Part model, mm, in its own coordinate system. Face numbers are marked on the shaded views. A direction names the side the tool comes from. Round coordinates to 2 decimals unless told otherwise and drop trailing zeros. Write each loop counter-clockwise with the first axis right and the second up, starting at its lowest first coordinate (ties: lowest second). Pieces come first, ordered by that corner, then holes.
1) Saw through at D-D on y = -22. Write the cut outline in (x, z) (1 decimal), and give its area (3 significant figures).
2) Saw through at A-A on y = -13. Write the cut outline in (x, z) (3 decimals), and give its area (3 significant figures).
3) Flat gauge pins, fed straight in: pin 1 (12 mm diameter, centred on x = 6, z = 12.5, fed in from +Y); pin 2 (8 mm diameter, centred on x = -4, z = 2, fed in from +Y); pin 3 (13 mm diameter, centred on x = -1, z = 3.5, fed in from +Y); pin 4 (8 mm diameter, centred on x = -6.5, z = -12.5, fed in from -Y). Where does each tip first touch, or does it go through?
4) Which spindle directions (+Z, -Z, +X, -X, +Y, -Y) get a long thin tool onto all of the face, cutting with end or side? Do the marked faces 4, 5 and 6. Say none if no direction does.
5) Drill centre lines: L1, parallel to Z at x = 12, y = 14.5 (3 decimals); L2, parallel to Z at x = 0, y = -28. Where is each one in solid material? Low to high.
6) Pull direction X, two halves, no side cores. Call the marked faces 1, 2 and 3: +X half, -X half, draft (parallel to the pull), parting line (faces both ways), or undercut.
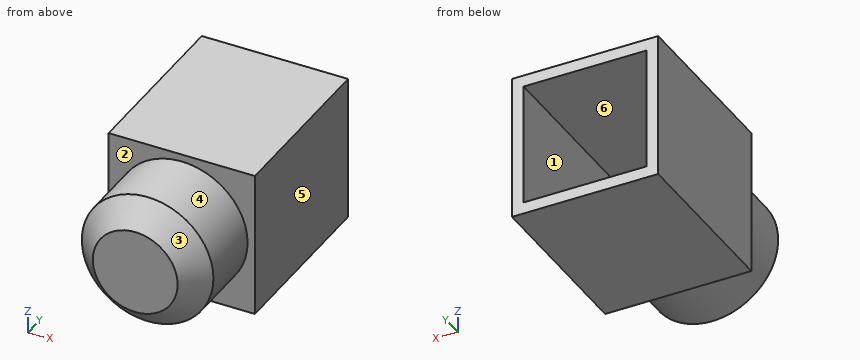
```python
from build123d import *

# Parameters (mm, degrees)
F0_W     = 31.75
F0_H     = 31.75
F1_DEPTH = 19.05
F2_R     = 14.2875
F3_DEPTH = 19.05
F4_SIZE  = 5.08
F5_T     = -2.54


with BuildPart() as f1:
    # F0 (on Front) → F1 (new body, symmetric)
    with BuildSketch(Plane.XZ):
        Rectangle(F0_W, F0_H)
    extrude(amount=F1_DEPTH, both=True)

    # F2 (on face) → F3 (join)
    with BuildSketch(Plane.XZ.offset(19.05)):
        Circle(F2_R)
    extrude(amount=F3_DEPTH)

    # F4
    f4_edges = [f1.edges().sort_by_distance(p)[0] for p in [
        (-14.2875, -38.1, 0),
    ]]
    chamfer(f4_edges, length=F4_SIZE)

    # F5
    f5_openings = [f1.faces().sort_by_distance(p)[0] for p in [
        (0, 19.05, 0),
    ]]
    offset(amount=F5_T, openings=f5_openings, kind=Kind.INTERSECTION)


solid = f1.part
```
Completed:
1. outline: circle Ø28.6 at (0, 0); hole circle Ø23.5 at (0, 0)
1. area: 208 mm2
2. outline: (-15.875, -15.875) - (15.875, -15.875) - (15.875, 15.875) - (-15.875, 15.875) - close; hole (-13.335, -13.335) - (13.335, -13.335) - (13.335, 13.335) - (-13.335, 13.335) - close
2. area: 297 mm2
3. pin 1: stops at y = 19.05
3. pin 2: stops at y = -35.24
3. pin 3: stops at y = -33.58
3. pin 4: stops at y = -37.22
4. face 4: -Y
4. face 5: +Z, -Z, +X, +Y, -Y
4. face 6: +Y
5. L1: z = -15.875 to -13.335, 13.335 to 15.875
5. L2: z = -14.29 to -11.75, 11.75 to 14.29
6. face 1: undercut
6. face 2: draft
6. face 3: parting line
